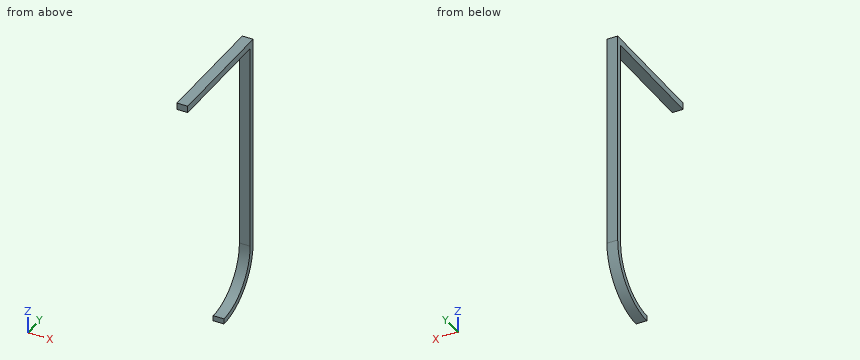
Autodesk Inventor part; units mm, degrees
ref_plane "YZ Plane" through (0, 0, 0) normal (1, 0, 0) x (0, 1, 0)
ref_plane "XZ Plane" through (0, 0, 0) normal (0, 1, 0) x (-1, 0, 0)
ref_plane "XY Plane" through (0, 0, 0) normal (0, 0, 1) x (1, 0, 0)
sketch "Sketch1" plane through (0, 0, 0) normal (1, 0, 0) x (0, 1, 0)
  line L0 (0, 10.0605) -> (0, 10.7499)
  arc A0 (0, -25.4) -> (25.4, 0) centre (0, 0) ccw
  arc A1 (0, -23.8125) -> (23.8125, 0) centre (0, 0) ccw
  line L1 (25.4, 0) -> (25.4, 101.6)
  line L2 (23.8125, 0) -> (23.8125, 101.6)
  line L3 (25.4, 101.6) -> (23.8125, 101.6)
  dimension "d2" = 25.4
  dimension "d3" = 101.6
  dimension "d4" = 101.6
extrude "Extrusion1" [suppressed]
sketch "Sketch2" plane through (0, 0, 0) normal (1, 0, 0) x (0, 1, 0)
  arc A0 (0, -25.4) -> (25.4, 0) centre (0, 0) ccw
  arc A1 (0, -22.86) -> (22.86, 0) centre (0, 0) ccw
  line L0 (0, -22.86) -> (0, -25.4)
  line L1 (25.4, 0) -> (25.4, 101.6)
  line L2 (22.86, 0) -> (22.86, 98.425)
  line L3 (22.86, 98.425) -> (-6.35, 98.425)
  line L4 (-6.35, 98.425) -> (-6.35, 101.6)
  line L5 (-6.35, 101.6) -> (14.2875, 101.6)
  line L6 (14.2875, 101.6) -> (16.1645, 101.6)
  line L7 (16.1645, 101.6) -> (25.4, 101.6)
  dimension "d5" = 25.4
  dimension "d6" = 22.86
  dimension "d8" = 101.6
extrude "Extrusion2" add sketch "Sketch2" along normal blind 5.08
sketch "Sketch3" plane through (0, -6.35, 98.425) normal (0, -1, 0) x (1, 0, 0)
  line L0 (5.08, -98.425) -> (5.08, 3.175)
  line L1 (0, 0) -> (5.08, 0)
  line L2 (5.08, 3.175) -> (0, 3.175)
  line L3 (0, 3.175) -> (0, 0)
  line L4 (0, 0) -> (5.08, 0)
  line L5 (5.08, 0) -> (5.08, 3.175)
  point P0 (0, -98.425)
extrude "Extrusion3" add sketch "Sketch3" along normal blind 25.4
properties part number "CONTAINER PIPE"
The listing builds one solid part. Answer for the finished solid, in the listing's coordinates (mm). Give positions to 0.01 mm unless a question says otherwise; leave off trailing zeros. Order: outer loops, then holes, each group sorted by start corner. A loop starts at its lowest first (then second) coordinate and runs counter-clockwise, first axis right, second up. Notation, with made-up numbers: (51, -26.75) -> (76, -26.75) arc R34 cw to (76, 9.25) -> close; hole circle Ø10 at (65, 5). An arc over 180 degrees is marked (long way). One line per item, written item: value.
1) Flat-ended cylindrical pins translate along their axes: P1, Ø3, axis at x = 1, z = 14.5, coming from the -Y side; P2, Ø3, axis at x = 3.5, z = -24.5, coming from the -Y side; P3, Ø3, axis at x = 1.5, z = -11, coming from the -Y side. Find the tip coordinate at first contact, or state that the pin passes through.
Reported:
P1: stops at y = 22.86
P2: stops at y = 0
P3: stops at y = 19.14
2) Find section D-D, the plane z = 20.5. Determine the outline of the cut face in (x, y), plus the area to 3 significant figures.
Reported:
outline: (0, 22.86) -> (5.08, 22.86) -> (5.08, 25.4) -> (0, 25.4) -> close
area: 12.9 mm^2
3) Find section A-A, the plane y = 14.5. Determine the outline of the cut face in (x, z) (1 decimal), plus the area to 3 significant figures.
Reported:
outline: (0, -20.9) -> (5.1, -20.9) -> (5.1, -17.7) -> (0, -17.7) -> close; (0, 98.4) -> (5.1, 98.4) -> (5.1, 101.6) -> (0, 101.6) -> close
area: 32.3 mm^2
4) Find section B-B, the plane x = 1.45. Determine the outline of the cut face in (y, z) (3 decimals).
Reported:
outline: (-31.75, 98.425) -> (22.86, 98.425) -> (22.86, 0) arc R22.86 cw to (0, -22.86) -> (0, -25.4) arc R25.4 ccw to (25.4, 0) -> (25.4, 101.6) -> (-31.75, 101.6) -> close
5) Find the intervals of material crossed by line 1 (Z direction, x = 3.7, y = 1) (3 decimals); line 2 (Y direction, x = 4.2, z = 21); line 3 (Z direction, x = 4.7, y = -10) (3 decimals), in increasing order.
Reported:
line 1: z = -25.38 to -22.838, 98.425 to 101.6
line 2: y = 22.86 to 25.4
line 3: z = 98.425 to 101.6
6) Find section C-C, the plane y = -3. Determine the outline of the cut face in (x, z) (3 decimals).
Reported:
outline: (0, 98.425) -> (5.08, 98.425) -> (5.08, 101.6) -> (0, 101.6) -> close
